Part model, mm, in its own coordinate system. A direction names the side the tool comes from. Round coordinates to 2 decimals unless told otherwise and drop trailing zeros. Write each loop counter-clockwise with the first axis right and the second up, starting at its lowest first coordinate (ties: lowest second). Pieces come first, ordered by that corner, then holes.
1) Pull direction X, two halves, no side cores. Call faces 1 (the cylindrical face through (44.594, 1.521, -28.719)), 2 (the flat face through (0, -5, 0)), 3 (the flat face through (-36, 1, 26.75)), 4 (the flat face through (36, 1, 18.25)): +X half, -X half, draft (parallel to the pull), parting line (faces both ways), or undercut.
2) Saw through at D-D on z = 0. Write the cut outline in (x, y).
3) Saw through at B-B on y = 1.25. Write the cut outline in (x, z).
4) Saw through at C-C on z = -24. Write the cut outline in (x, y), and give its area (3 significant figures).
5) Which spindle directions (+Z, -Z, +X, -X, +Y, -Y) get a long thin tool onto all of the face, cutting with end or side? Do faces 5 (the cylindrical face through (-30.75, 1.48, -22.59)), 6 (the flat face through (-1, 3, 0)). Say none if no direction does.
6) Drill centre lines: L1, parallel to X at y = 2, z = 20; L2, parallel to Y at x = -25.5, z = -19.5; L3, parallel to X at y = -0.5, z = -13.5. Where is each one in solid material? Low to high.
7) Saw through at A-A on x = -24. Write the cut outline in (y, z).
```python
from build123d import *

# Parameters (mm, degrees)
SKETCH_1_W      = 94
SKETCH_1_H      = 62
EXTRUDE_1_DEPTH = 3
FILLET_1_R      = 8
SKETCH_7_R      = 30
EXTRUDE_2_DEPTH = 5


with BuildPart() as part:
    # 草图1 → 凸台-拉伸1 (new body)
    with BuildSketch(Plane(origin=(0, 0, 0), x_dir=(1, 0, 0), z_dir=(0, 1, 0))):
        Rectangle(SKETCH_1_W, SKETCH_1_H)
        with BuildLine():
            Line((-37, 26.75), (-35, 26.75))
            ThreePointArc((-35, 26.75), (-30.75, 22.5), (-35, 18.25))
            Line((-35, 18.25), (-37, 18.25))
            ThreePointArc((-37, 18.25), (-41.25, 22.5), (-37, 26.75))
        make_face(mode=Mode.SUBTRACT)
        with BuildLine():
            Line((37, 26.75), (35, 26.75))
            ThreePointArc((35, 26.75), (30.75, 22.5), (35, 18.25))
            Line((35, 18.25), (37, 18.25))
            ThreePointArc((37, 18.25), (41.25, 22.5), (37, 26.75))
        make_face(mode=Mode.SUBTRACT)
        with BuildLine():
            Line((37, -26.75), (35, -26.75))
            ThreePointArc((35, -26.75), (30.75, -22.5), (35, -18.25))
            Line((35, -18.25), (37, -18.25))
            ThreePointArc((37, -18.25), (41.25, -22.5), (37, -26.75))
        make_face(mode=Mode.SUBTRACT)
        with BuildLine():
            Line((-37, -26.75), (-35, -26.75))
            ThreePointArc((-35, -26.75), (-30.75, -22.5), (-35, -18.25))
            Line((-35, -18.25), (-37, -18.25))
            ThreePointArc((-37, -18.25), (-41.25, -22.5), (-37, -26.75))
        make_face(mode=Mode.SUBTRACT)
    extrude(amount=EXTRUDE_1_DEPTH)

    # 圆角1
    fillet_1_edges = [part.edges().sort_by_distance(p)[0] for p in [
        (-47, 1.5, -31),
        (47, 1.5, -31),
        (47, 1.5, 31),
        (-47, 1.5, 31),
    ]]
    fillet(fillet_1_edges, radius=FILLET_1_R)

    # 草图7 → 凸台-拉伸2 (add)
    with BuildSketch(Plane.XZ):
        with Locations(Location((0, 0, 0), (0, 0, 90))):
            Circle(SKETCH_7_R)
    extrude(amount=EXTRUDE_2_DEPTH)


solid = part.part
```
Completed:
1. face 1: +X half
1. face 2: draft
1. face 3: undercut
1. face 4: undercut
2. outline: (-47, 0) - (-30, 0) - (-30, -5) - (30, -5) - (30, 0) - (47, 0) - (47, 3) - (-47, 3) - close
3. outline: (-47, -23) arc R8 ccw to (-39, -31) - (39, -31) arc R8 ccw to (47, -23) - (47, 23) arc R8 ccw to (39, 31) - (-39, 31) arc R8 ccw to (-47, 23) - close; hole (-37, -26.75) - (-35, -26.75) arc R4.25 ccw to (-35, -18.25) - (-37, -18.25) arc R4.25 ccw to start; hole (-37, 18.25) - (-35, 18.25) arc R4.25 ccw to (-35, 26.75) - (-37, 26.75) arc R4.25 ccw to start; hole (35, -26.75) - (37, -26.75) arc R4.25 ccw to (37, -18.25) - (35, -18.25) arc R4.25 ccw to start; hole (35, 18.25) - (37, 18.25) arc R4.25 ccw to (37, 26.75) - (35, 26.75) arc R4.25 ccw to start
4. outline: (-46.94, 0) - (-40.98, 0) - (-40.98, 3) - (-46.94, 3) - close; (-31.02, 0) - (-18, 0) - (-18, -5) - (18, -5) - (18, 0) - (31.02, 0) - (31.02, 3) - (-31.02, 3) - close; (40.98, 0) - (46.94, 0) - (46.94, 3) - (40.98, 3) - close
4. area: 402 mm2
5. face 5: +Y, -Y
5. face 6: +Z, -Z, +X, -X, +Y
6. L1: x = -47 to -40.44, -31.56 to 31.56, 40.44 to 47
6. L2: y = 0 to 3
6. L3: x = -26.79 to 26.79
7. outline: (-5, -18) - (0, -18) - (0, -31) - (3, -31) - (3, 31) - (0, 31) - (0, 18) - (-5, 18) - close
